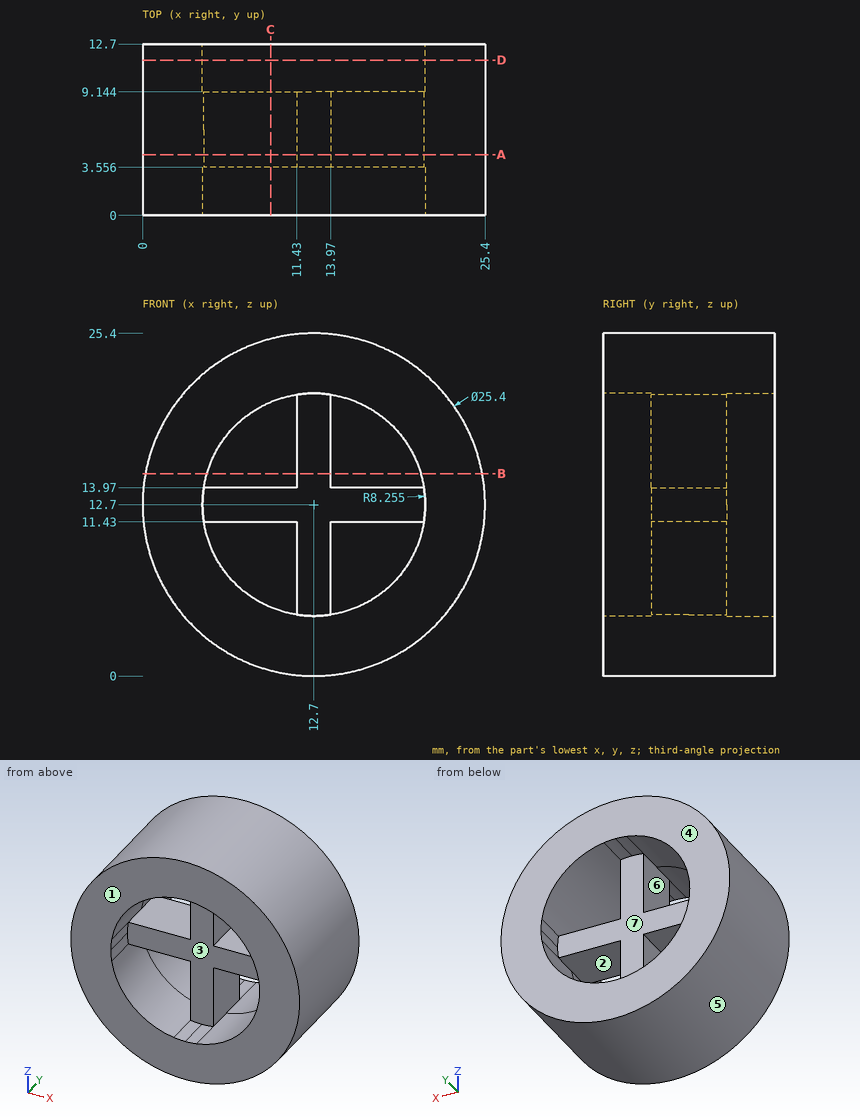
Input: dimensioned drawing with shaded views. Units: mm. Origin: part minimum x, y, z. A direction names the side the tool comes from. Give positions to 0.01 mm unless a question says otherwise; leave off trailing zeros. Loops run counter-clockwise (first coordinate to the right, second up) from the corner with the lowest first, then second, coordinate; pieces in that order, holes last. Notation, with made-up numbers: M 52,66 L 98,66 A22 cw 98,80 Z; hole C -24.5,60.5 d9. An arc over 180 degrees is marked long. Put each result on its own line as item: value. Start each with the question number.
1) Cut plane C-C (x = 9.5). Output: boundary loops of the cut face in (y, z), then the cut area to 3 significant figures.
2) Pull-direction query (Z, two-part tool) for the marked faces 4, 5, 6 and 7; classes: pulls with the +Z half, pulls with the -Z half, needs draft (parallel to the pull), parting line crosses it, or undercut.
3) Cut plane B-B (z = 15). Output: boundary loops of the cut face in (x, y), then the cut area to 3 significant figures.
4) Access query for the marked faces 1, 2 and 3. Directions: +Z, -Z, +X, -X, +Y, -Y. A direction counts if a zero-diameter tool reaches every point of the face in a straight line with its end or side. Return the directions, or none.
5) Ray query, line 1 along X through (y, z) = (4.25, 8); line 2 along X through (y, z) = (4.5, 15); line 3 along Z through (x, y) = (16.75, 3.75). Return the intervals inside material, ascending.
6) Cut plane D-D (y = 11.5). Output: boundary loops of the cut face in (x, z) (3 decimals).
7) Contact query for flat-ended pins moving along their axis: pin 1 (5 mm diameter, centred on x = 20.5, y = 9.5, fed in from -Z); pin 2 (2 mm diameter, centred on x = 15, y = 2, fed in from -Z); pin 3 (3 mm diameter, centred on x = 19, y = 6, fed in from +Z); pin 4 (13 mm diameter, centred on x = 11, z = 10, fed in from +Y). Output: stop coordinate, or through.
8) Cut plane A-A (y = 4.5). Output: boundary loops of the cut face in (x, z) (3 decimals).
Verdict:
1. outline: M 0,0.41 L 12.7,0.41 L 12.7,5.09 L 0,5.09 Z; M 0,20.31 L 12.7,20.31 L 12.7,24.99 L 0,24.99 Z; M 3.56,11.43 L 9.14,11.43 L 9.14,13.97 L 3.56,13.97 Z
1. area: 133 mm2
2. face 4: needs draft
2. face 5: parting line crosses it
2. face 6: undercut
2. face 7: undercut
3. outline: M 0.21,0 L 4.77,0 L 4.77,12.7 L 0.21,12.7 Z; M 11.43,3.56 L 13.97,3.56 L 13.97,9.14 L 11.43,9.14 Z; M 20.63,0 L 25.19,0 L 25.19,12.7 L 20.63,12.7 Z
3. area: 130 mm2
4. face 1: +Z, -Z, +X, -X, -Y
4. face 2: +Y, -Y
4. face 3: -Y
5. line 1: 0.9 to 5.91, 11.43 to 13.97, 19.49 to 24.5
5. line 2: 0.21 to 4.77, 11.43 to 13.97, 20.63 to 25.19
5. line 3: 0.66 to 5.51, 11.43 to 13.97, 19.89 to 24.74
6. outline: C 12.7,12.7 d25.4; hole C 12.7,12.7 d16.51
7. pin 1: z = 1.16
7. pin 2: z = 0.07
7. pin 3: z = 24.46
7. pin 4: y = 12.7
8. outline: C 12.7,12.7 d25.4; hole M 4.543,11.43 A8.255 ccw 11.43,4.543 L 11.43,11.43 Z; hole M 4.543,13.97 L 11.43,13.97 L 11.43,20.857 A8.255 ccw Z; hole M 13.97,4.543 A8.255 ccw 20.857,11.43 L 13.97,11.43 Z; hole M 13.97,13.97 L 20.857,13.97 A8.255 ccw 13.97,20.857 Z
